Could you check a few things on this model? Use its own coordinates, in mm. A direction names the side the tool comes from. Round coordinates to 2 decimals unless told otherwise and drop trailing zeros. Order: outer loops, then holes, each group sorted by start corner. A loop starts at its lowest first (then second) coordinate and runs counter-clockwise, first axis right, second up. Notation, with made-up numbers: M -15.75,23 L -6.75,23 A22 cw -6.75,57 Z; hole C 15.5,0 d2. An arc over 180 degrees is marked long. Write each question's results on one line, items separated by ' | '. Start each with the question number.
1. Suppose I cut it at A-A on x = -14. Write out the boundary of the cut face in (y, z).
2. We'd pull the mould along Z, two halves only. Please class faces 4 (the flat face through (0, -13, 0)), 5 (the cylindrical face through (-10.59, -1.01, -2.31)), 6 (the flat face through (-13, -1, -7.5)): released by +Z, released by -Z, zero draft, split by the parting line, or undercut.
3. Please list where these lines run through material, in increasing order: L1, parallel to Y at x = -2.5, z = 4.75; L2, parallel to Z at x = -8.75, y = -12.25; L3, parallel to Z at x = -3.5, y = -8.5.
4. For faces 1 (the flat face through (3.451, -0.986, -7.458)), 2 (the flat face through (-4.5, -6.6, 10)), 3 (the flat face through (0, -6, 9)), which set-ups out of +Z, -Z, +X, -X, +Y, -Y let a thin tool reach every point of the face, with its end or its side?
5. I'm going to push flat-ended pins straight in: pin 1 (0.6 mm diameter, centred on y = -7, z = 9.5, fed in from -X); pin 2 (2 mm diameter, centred on x = -12, y = -12.5, fed in from +Z); pin 3 (2 mm diameter, centred on x = -1, y = -7.5, fed in from -Z). Where does each tip first touch, or does it pass through?
6. Suppose I cut it at C-C on z = -8.25. Write out the boundary of the cut face in (x, y), and give its area (3 significant figures).
7. Suppose I cut it at B-B on x = 8.75. Write out the boundary of the cut face in (y, z).
from build123d import *

# Parameters (mm, degrees)
F0_W      = 33
F0_H      = 22
F2_DEPTH  = 13
F3_SIZE   = 7
F4_R      = 2.5
F5_DEPTH  = 25
F6_T      = -2
F7_W      = 11
F7_H      = 13
F8_DEPTH  = 2
F9_SIZE   = 1.99999
F11_DEPTH = 25
F12_SIZE  = 2


# Not quite as in the source:
# - a fillet or chamfer is up to 0.001 mm smaller than in the source, because OpenCascade refuses the exact size


with BuildPart() as f2:
    # F0 (on Front) → F2 (new body)
    with BuildSketch(Plane.XZ):
        Rectangle(F0_W, F0_H)
    extrude(amount=F2_DEPTH)

    # F3
    f3_edges = [f2.edges().sort_by_distance(p)[0] for p in [
        (-16.5, -6.5, -11),
        (16.5, -6.5, -11),
    ]]
    chamfer(f3_edges, length=F3_SIZE)

    # F4 (on face) → F5 (cut)
    with BuildSketch(Plane.XZ.offset(13)):
        with Locations((-8.75, -4)):
            Circle(F4_R)
        with Locations((8.75, -4)):
            Circle(F4_R)
    extrude(amount=-F5_DEPTH, mode=Mode.SUBTRACT)

    # F6
    f6_openings = [f2.faces().sort_by_distance(p)[0] for p in [
        (0, -6.5, -11),
        (13, -6.5, -7.5),
        (16.5, -6.5, 3.5),
        (-16.5, -6.5, 3.5),
        (-13, -6.5, -7.5),
        (-11.25, -6.5, -4),
        (6.25, -6.5, -4),
    ]]
    offset(amount=F6_T, openings=f6_openings)

    # F7 (on face) → F8 (cut)
    with BuildSketch(Plane.XY.offset(11)):
        with Locations((11, -6.5)):
            Rectangle(F7_W, F7_H)
        with Locations((-11, -6.5)):
            Rectangle(F7_W, F7_H)
    extrude(amount=-F8_DEPTH, mode=Mode.SUBTRACT)

    # F9 (size 2 in the source; OpenCascade refuses exactly that, so slightly less here)
    f9_edges = [f2.edges().sort_by_distance(p)[0] for p in [
        (5.5, -6.5, 9),
        (-5.5, -6.5, 9),
    ]]
    chamfer(f9_edges, length=F9_SIZE)

    # F10 (on face) → F11 (cut)
    with BuildSketch(Plane(origin=(0, 0, 0), x_dir=(-1, 0, 0), z_dir=(0, 1, 0))):
        Polygon((7, -11), (0, -4.0134343201), (-7, -11), align=None)
    extrude(amount=-F11_DEPTH, mode=Mode.SUBTRACT)

    # F12
    f12_edges = [f2.edges().sort_by_distance(p)[0] for p in [
        (16.5, -12, 9),
        (16.5, -1, 9),
        (-16.5, -12, 9),
        (-16.5, -1, 9),
    ]]
    chamfer(f12_edges, length=F12_SIZE)


solid = f2.part
Filled sheet:
1) outline: M -13,-6.5 L -11,-6.5 L -11,9 L -13,9 Z; M -2,-6.5 L 0,-6.5 L 0,9 L -2,9 Z
2) face 4: zero draft | face 5: undercut | face 6: released by -Z
3) L1: y = -13 to -11, -2 to 0 | L2: z = -11 to -6.5, -1.5 to 9 | L3: z = 9 to 11
4) face 1: -Z, +Y, -Y | face 2: -Z, -X | face 3: -Z, +X, -X
5) pin 1: stops at x = -4.3 | pin 2: stops at z = 9 | pin 3: stops at z = 9
6) outline: M -12.25,-13 L -4.24,-13 L -4.24,-11 L -12.25,-11 Z; M -12.25,-2 L -4.24,-2 L -4.24,0 L -12.25,0 Z; M 4.24,-13 L 12.25,-13 L 12.25,-11 L 4.24,-11 Z; M 4.24,-2 L 12.25,-2 L 12.25,0 L 4.24,0 Z | area: 64.0 mm^2
7) outline: M -13,-11 L -11,-11 L -11,-6.5 L -13,-6.5 Z; M -13,-1.5 L -11,-1.5 L -11,9 L -13,9 Z; M -2,-11 L 0,-11 L 0,-6.5 L -2,-6.5 Z; M -2,-1.5 L 0,-1.5 L 0,9 L -2,9 Z
